Could you check a few things on this model? Use its own coordinates, in mm. A direction names the side the tool comes from. Give positions to 0.01 mm unless a question says otherwise; leave off trailing zeros. Loops run counter-clockwise (first coordinate to the right, second up) from the corner with the lowest first, then second, coordinate; pieces in that order, holes last. Notation, with made-up numbers: (-36.75, -31) - (-9.75, -31) arc R32 ccw to (-9.75, 5) - close; hole circle Ø7 at (54, -30). An arc over 180 degrees is marked (long way). Use CSV: the item, a comma, the result in double quotes.
from build123d import *

# Parameters (mm, degrees)
ESQUISSE1_R             = 5
ESQUISSE1_R_2           = 10
BOSS_EXTRU_1_DEPTH      = 10
CONG_1_R                = 2
ENL_V_MAT_EXTRU_1_DEPTH = 1


with BuildPart() as part:
    # Esquisse1 → Boss.-Extru.1 (new body)
    # profile 1 of 19: a face of its own
    with BuildSketch(Plane(origin=(0, 0, 0), x_dir=(0, 1, 0), z_dir=(0, 0, 1))):
        with Locations((0, -29)):
            Circle(ESQUISSE1_R)
    # profile 2 of 19: a face of its own
    with BuildSketch(Plane(origin=(0, 0, 0), x_dir=(0, 1, 0), z_dir=(0, 0, 1))):
        with BuildLine():
            ThreePointArc((5.99413543, -10.382147113), (3.146801004, -10.052477503), (0.281000689, -9.996051151))
            ThreePointArc((0.281000689, -9.996051151), (0, -10), (-0.281000689, -9.996051151))
            ThreePointArc((-0.281000689, -9.996051151), (-3.146801004, -10.052477503), (-5.99413543, -10.382147113))
            ThreePointArc((-5.99413543, -10.382147113), (-4.127637704, -19.033097235), (-4.866476509, -27.852216749))
            ThreePointArc((-4.866476509, -27.852216749), (0, -24), (4.866476509, -27.852216749))
            ThreePointArc((4.866476509, -27.852216749), (4.127637704, -19.033097235), (5.99413543, -10.382147113))
        make_face()
    # profile 3 of 19: a face of its own
    with BuildSketch(Plane(origin=(0, 0, 0), x_dir=(0, 1, 0), z_dir=(0, 0, 1))):
        with Locations((25.11473671, -14.5)):
            Circle(ESQUISSE1_R)
    # profile 4 of 19: a face of its own
    with BuildSketch(Plane(origin=(0, 0, 0), x_dir=(0, 1, 0), z_dir=(0, 0, 1))):
        with BuildLine():
            ThreePointArc((11.98827086, 0), (10.279101391, -2.301029141), (8.797334579, -4.754671841))
            ThreePointArc((8.797334579, -4.754671841), (8.660254038, -5), (8.51633389, -5.24137931))
            ThreePointArc((8.51633389, -5.24137931), (7.132300386, -7.751448362), (5.99413543, -10.382147113))
            ThreePointArc((5.99413543, -10.382147113), (14.419326866, -13.091187726), (21.687489002, -18.140600658))
            ThreePointArc((21.687489002, -18.140600658), (20.784609691, -12), (26.55396551, -9.711616091))
            ThreePointArc((26.55396551, -9.711616091), (18.54696457, -5.941909508), (11.98827086, 0))
        make_face()
    # profile 5 of 19: a face of its own
    with BuildSketch(Plane(origin=(0, 0, 0), x_dir=(0, 1, 0), z_dir=(0, 0, 1))):
        with Locations((-25.11473671, -14.5)):
            Circle(ESQUISSE1_R)
    # profile 6 of 19: a face of its own
    with BuildSketch(Plane(origin=(0, 0, 0), x_dir=(0, 1, 0), z_dir=(0, 0, 1))):
        with BuildLine():
            ThreePointArc((-5.99413543, -10.382147113), (-7.132300386, -7.751448362), (-8.51633389, -5.24137931))
            ThreePointArc((-8.51633389, -5.24137931), (-8.660254038, -5), (-8.797334579, -4.754671841))
            ThreePointArc((-8.797334579, -4.754671841), (-10.279101391, -2.301029141), (-11.98827086, 0))
            ThreePointArc((-11.98827086, 0), (-18.54696457, -5.941909508), (-26.55396551, -9.711616091))
            ThreePointArc((-26.55396551, -9.711616091), (-22.131126816, -10.487759728), (-20.11473671, -14.5))
            ThreePointArc((-20.11473671, -14.5), (-20.524734611, -16.482897055), (-21.687489002, -18.140600658))
            ThreePointArc((-21.687489002, -18.140600658), (-14.419326866, -13.091187726), (-5.99413543, -10.382147113))
        make_face()
    # profile 7 of 19: a face of its own
    with BuildSketch(Plane(origin=(0, 0, 0), x_dir=(0, 1, 0), z_dir=(0, 0, 1))):
        with BuildLine():
            ThreePointArc((-8.797334579, 4.754671841), (-8.660254038, 5), (-8.51633389, 5.24137931))
            ThreePointArc((-8.51633389, 5.24137931), (-7.132300386, 7.751448362), (-5.99413543, 10.382147113))
            ThreePointArc((-5.99413543, 10.382147113), (-14.419326866, 13.091187726), (-21.687489002, 18.140600658))
            ThreePointArc((-21.687489002, 18.140600658), (-20.524734611, 16.482897055), (-20.11473671, 14.5))
            ThreePointArc((-20.11473671, 14.5), (-22.131126816, 10.487759728), (-26.55396551, 9.711616091))
            ThreePointArc((-26.55396551, 9.711616091), (-18.54696457, 5.941909508), (-11.98827086, 0))
            ThreePointArc((-11.98827086, 0), (-10.279101391, 2.301029141), (-8.797334579, 4.754671841))
        make_face()
    # profile 8 of 19: a face of its own
    with BuildSketch(Plane(origin=(0, 0, 0), x_dir=(0, 1, 0), z_dir=(0, 0, 1))):
        with Locations((-25.11473671, 14.5)):
            Circle(ESQUISSE1_R)
    # profile 9 of 19: a face of its own
    with BuildSketch(Plane(origin=(0, 0, 0), x_dir=(0, 1, 0), z_dir=(0, 0, 1))):
        with BuildLine():
            ThreePointArc((-8.797334579, -4.754671841), (-10, 0), (-8.797334579, 4.754671841))
            ThreePointArc((-8.797334579, 4.754671841), (-10.279101391, 2.301029141), (-11.98827086, 0))
            ThreePointArc((-11.98827086, 0), (-10.279101391, -2.301029141), (-8.797334579, -4.754671841))
        make_face()
    # profile 10 of 19: a face of its own
    with BuildSketch(Plane(origin=(0, 0, 0), x_dir=(0, 1, 0), z_dir=(0, 0, 1))):
        with BuildLine():
            ThreePointArc((-5.99413543, -10.382147113), (-3.146801004, -10.052477503), (-0.281000689, -9.996051151))
            ThreePointArc((-0.281000689, -9.996051151), (-5, -8.660254038), (-8.51633389, -5.24137931))
            ThreePointArc((-8.51633389, -5.24137931), (-7.132300386, -7.751448362), (-5.99413543, -10.382147113))
        make_face()
    # profile 11 of 19: a face of its own
    with BuildSketch(Plane(origin=(0, 0, 0), x_dir=(0, 1, 0), z_dir=(0, 0, 1))):
        Circle(ESQUISSE1_R_2)
        Polygon((4.8, 2.771281292), (0, 5.542562584), (-4.8, 2.771281292), (-4.8, -2.771281292), (0, -5.542562584), (4.8, -2.771281292), align=None, mode=Mode.SUBTRACT)
    # profile 12 of 19: a face of its own
    with BuildSketch(Plane(origin=(0, 0, 0), x_dir=(0, 1, 0), z_dir=(0, 0, 1))):
        with BuildLine():
            ThreePointArc((-8.51633389, 5.24137931), (-5, 8.660254038), (-0.281000689, 9.996051151))
            ThreePointArc((-0.281000689, 9.996051151), (-3.146801004, 10.052477503), (-5.99413543, 10.382147113))
            ThreePointArc((-5.99413543, 10.382147113), (-7.132300386, 7.751448362), (-8.51633389, 5.24137931))
        make_face()
    # profile 13 of 19: a face of its own
    with BuildSketch(Plane(origin=(0, 0, 0), x_dir=(0, 1, 0), z_dir=(0, 0, 1))):
        with BuildLine():
            ThreePointArc((-0.281000689, 9.996051151), (0, 10), (0.281000689, 9.996051151))
            ThreePointArc((0.281000689, 9.996051151), (3.146801004, 10.052477503), (5.99413543, 10.382147113))
            ThreePointArc((5.99413543, 10.382147113), (4.127637704, 19.033097235), (4.866476509, 27.852216749))
            ThreePointArc((4.866476509, 27.852216749), (0, 24), (-4.866476509, 27.852216749))
            ThreePointArc((-4.866476509, 27.852216749), (-4.127637704, 19.033097235), (-5.99413543, 10.382147113))
            ThreePointArc((-5.99413543, 10.382147113), (-3.146801004, 10.052477503), (-0.281000689, 9.996051151))
        make_face()
    # profile 14 of 19: a face of its own
    with BuildSketch(Plane(origin=(0, 0, 0), x_dir=(0, 1, 0), z_dir=(0, 0, 1))):
        with BuildLine():
            ThreePointArc((8.51633389, 5.24137931), (8.660254038, 5), (8.797334579, 4.754671841))
            ThreePointArc((8.797334579, 4.754671841), (10.279101391, 2.301029141), (11.98827086, 0))
            ThreePointArc((11.98827086, 0), (18.54696457, 5.941909508), (26.55396551, 9.711616091))
            ThreePointArc((26.55396551, 9.711616091), (20.784609691, 12), (21.687489002, 18.140600658))
            ThreePointArc((21.687489002, 18.140600658), (14.419326866, 13.091187726), (5.99413543, 10.382147113))
            ThreePointArc((5.99413543, 10.382147113), (7.132300386, 7.751448362), (8.51633389, 5.24137931))
        make_face()
    # profile 15 of 19: a face of its own
    with BuildSketch(Plane(origin=(0, 0, 0), x_dir=(0, 1, 0), z_dir=(0, 0, 1))):
        with BuildLine():
            ThreePointArc((0.281000689, 9.996051151), (5, 8.660254038), (8.51633389, 5.24137931))
            ThreePointArc((8.51633389, 5.24137931), (7.132300386, 7.751448362), (5.99413543, 10.382147113))
            ThreePointArc((5.99413543, 10.382147113), (3.146801004, 10.052477503), (0.281000689, 9.996051151))
        make_face()
    # profile 16 of 19: a face of its own
    with BuildSketch(Plane(origin=(0, 0, 0), x_dir=(0, 1, 0), z_dir=(0, 0, 1))):
        with BuildLine():
            ThreePointArc((8.797334579, 4.754671841), (9.694672397, 2.452208618), (10, 0))
            ThreePointArc((10, 0), (9.694672397, -2.452208618), (8.797334579, -4.754671841))
            ThreePointArc((8.797334579, -4.754671841), (10.279101391, -2.301029141), (11.98827086, 0))
            ThreePointArc((11.98827086, 0), (10.279101391, 2.301029141), (8.797334579, 4.754671841))
        make_face()
    # profile 17 of 19: a face of its own
    with BuildSketch(Plane(origin=(0, 0, 0), x_dir=(0, 1, 0), z_dir=(0, 0, 1))):
        with BuildLine():
            ThreePointArc((5.99413543, -10.382147113), (7.132300386, -7.751448362), (8.51633389, -5.24137931))
            ThreePointArc((8.51633389, -5.24137931), (5, -8.660254038), (0.281000689, -9.996051151))
            ThreePointArc((0.281000689, -9.996051151), (3.146801004, -10.052477503), (5.99413543, -10.382147113))
        make_face()
    # profile 18 of 19: a face of its own
    with BuildSketch(Plane(origin=(0, 0, 0), x_dir=(0, 1, 0), z_dir=(0, 0, 1))):
        with Locations((25.11473671, 14.5)):
            Circle(ESQUISSE1_R)
    # profile 19 of 19: a face of its own
    with BuildSketch(Plane(origin=(0, 0, 0), x_dir=(0, 1, 0), z_dir=(0, 0, 1))):
        with Locations((0, 29)):
            Circle(ESQUISSE1_R)
    extrude(amount=BOSS_EXTRU_1_DEPTH)

    # Congé1
    cong_1_edges = [part.edges().sort_by_distance(p)[0] for p in [
        (10.382147113, 5.99413543, 5),
        (10.382147113, -5.99413543, 5),
        (0, -11.98827086, 5),
        (-10.382147113, -5.99413543, 5),
        (-10.382147113, 5.99413543, 5),
        (0, 11.98827086, 5),
    ]]
    fillet(cong_1_edges, radius=CONG_1_R)

    # Esquisse2 → Enlèv. mat.-Extru.1 (cut)
    with BuildSketch(Plane(origin=(0, 0, 0), x_dir=(1, 0, 0), z_dir=(0, 0, -1))):
        with BuildLine():
            Line((0, 9.5), (-2, 8.261355821))
            Line((-2, 8.261355821), (0, 7.5))
            ThreePointArc((0, 7.5), (5.303300859, -5.303300859), (-7.5, 0))
            Line((-7.5, 0), (-8.261355821, -2))
            Line((-8.261355821, -2), (-9.5, 0))
            ThreePointArc((-9.5, 0), (6.717514421, -6.717514421), (0, 9.5))
        make_face()
        Polygon((-7.471570722, 6.176220416), (-7.471570722, 7.394169134), (-6.638237388, 7.394169134), (-6.638237388, 6.176220416), (-5.356186106, 6.176220416), (-5.356186106, 5.342887082), (-6.638237388, 5.342887082), (-6.638237388, 4.124938365), (-7.471570722, 4.124938365), (-7.471570722, 5.342887082), (-8.753622004, 5.342887082), (-8.753622004, 6.176220416), align=None)
    extrude(amount=-ENL_V_MAT_EXTRU_1_DEPTH, mode=Mode.SUBTRACT)


solid = part.part
1) Suppose I cut it at A-A (x = 14.5). Please give me the cut outline in (y, z), plus the area to 3 significant figures.
Answer below:
outline,"(-30.11, 0) - (-16.95, 0) - (-16.95, 10) - (-30.11, 10) - close; (-4.77, 0) - (4.77, 0) - (4.77, 10) - (-4.77, 10) - close; (16.95, 0) - (30.11, 0) - (30.11, 10) - (16.95, 10) - close"
area,"359 mm2"
2) Suppose I cut it at D-D (y = 18.5). Please give me the cut outline in (x, z).
Answer below:
outline,"(-15.53, 0) - (-5.91, 0) - (-5.91, 10) - (-15.53, 10) - close; (5.91, 0) - (15.53, 0) - (15.53, 10) - (5.91, 10) - close"
3) I'm going to push flat-ended pins straight in: P1, Ø4.5, axis at x = 0, z = 3, coming from the -Y side; P2, Ø0.8, axis at x = -8, z = 0.5, coming from the -Y side; P3, Ø3, axis at y = -6, z = 2.5, coming from the +X side. Where does each tip first touch, or does it pass through?
Answer below:
P1,"stops at y = -14.03"
P2,"stops at y = -23.01"
P3,"stops at x = 31.18"
4) I need wall thicknesses on line 1 along X through (y, z) = (-0.5, 8); line 2 along Y through (x, z) = (-12.5, 3); line 3 along X through (y, z) = (-18.5, 9.5). Which ranges of each line are inside material? Lowest first, please.
Answer below:
line 1,"x = -33.97 to -5.25, 5.25 to 33.97"
line 2,"y = -29.7 to -13.15, -5.28 to 5.28, 13.15 to 29.7"
line 3,"x = -15.53 to -5.91, 5.91 to 15.53"
5) Which directions (+Z, -Z, +X, -X, +Y, -Y) give clear straight access to the entire face, cutting with the end or side of a thin tool? Please do faces 1 (the cylindrical face through (13.555, -15.319, 4.93)), 2 (the flat face through (0, -4.8, 5)), 3 (the cylindrical face through (6.37, -19.21, 4.93)), 4 (the cylindrical face through (-13.555, 15.319, 4.93)).
Answer below:
face 1,"+Z, -Z, +X"
face 2,"+Z, -Z"
face 3,"+Z, -Z, -Y"
face 4,"+Z, -Z, -X"
6) We'd pull the mould along X, two halves only. Please class faces 5 (the cylindrical face through (-13.45, -15.12, 4.93)), 6 (the cylindrical face through (6.49, 19.4, 4.93)), 7 (the flat face through (-4.14, 2.43, 4.93)), 8 (the flat face through (0, 7, 10)): +X half, -X half, draft (parallel to the pull), parting line (faces both ways), or undercut.
Answer below:
face 5,"-X half"
face 6,"undercut"
face 7,"undercut"
face 8,"draft"
7) Suppose I cut it at C-C (x = 29). Please give me the cut outline in (y, z), plus the area to 3 significant figures.
Answer below:
outline,"(-5, 0) - (5, 0) - (5, 10) - (-5, 10) - close"
area,"100 mm2"
8) Suppose I cut it at B-B (y = -1). Please give me the cut outline in (x, z), plus the area to 3 significant figures.
Answer below:
outline,"(-33.9, 0) - (-4.97, 0) - (-4.97, 10) - (-33.9, 10) - close; (4.97, 0) - (7.43, 0) - (7.43, 1) - (9.45, 1) - (9.45, 0) - (33.9, 0) - (33.9, 10) - (4.97, 10) - close"
area,"577 mm2"
